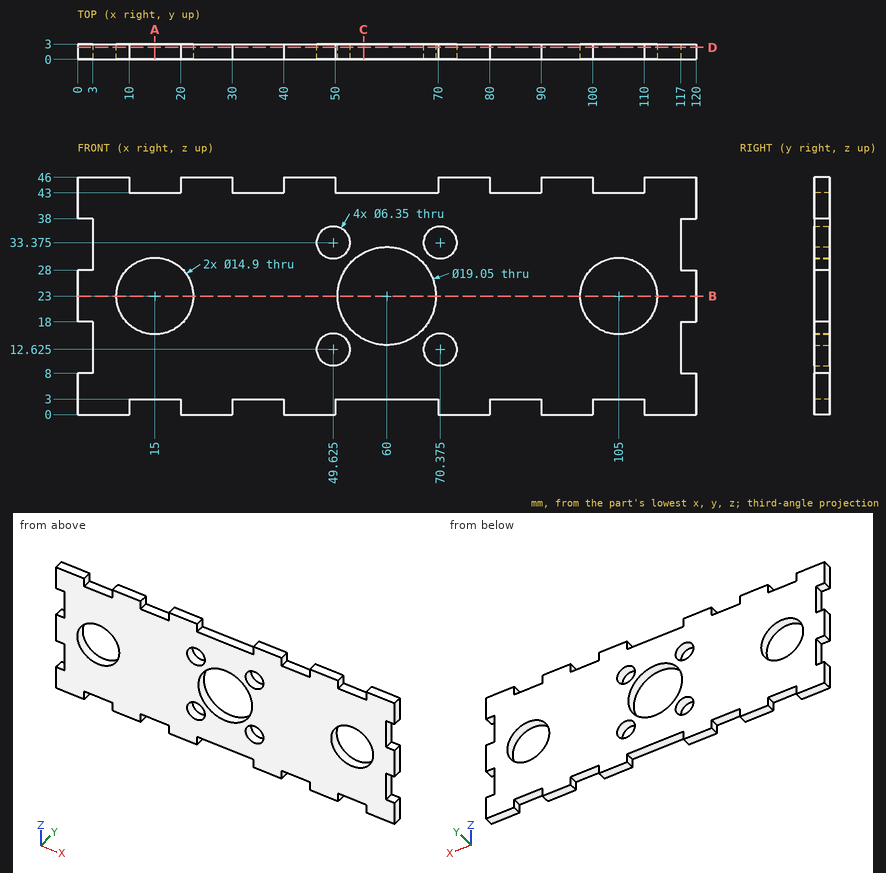
Drawing for the job (mm, zero at the part's lowest x, y, z). Coordinates: 2 decimals unless noted, no trailing zeros. Order: outer loops, then holes, each group sorted by start corner. A loop starts at its lowest first (then second) coordinate and runs counter-clockwise, first axis right, second up. Notation, with made-up numbers: (85, 66) -> (103, 66) arc R34 cw to (103, 102) -> close; hole circle Ø8 at (22.25, -3.5). An arc over 180 degrees is marked (long way). Return JSON: item names as keys, results as strings.
Item 1: Wall check: line 1 along X through (y, z) = (0.9, 23.5); line 2 along Z through (x, y) = (15, 1.1); line 3 along X through (y, z) = (1.45, 17.5). Give the ranges that are in metal, low to high. Write a range as from..to.
Model answer:
{"line 1": "x = 0..7.57, 22.43..50.49, 69.51..97.57, 112.43..120", "line 2": "z = 3..15.55, 30.45..43", "line 3": "x = 3..9.97, 20.03..52.22, 67.78..99.97, 110.03..117"}
Item 2: Slice it at B-B (z = 23). Write the cut outline in (x, y) (3 decimals), then the cut area to 3 significant figures.
Model answer:
{"outline": "(0, 0) -> (7.55, 0) -> (7.55, 3) -> (0, 3) -> close; (22.45, 0) -> (50.475, 0) -> (50.475, 3) -> (22.45, 3) -> close; (69.525, 0) -> (97.55, 0) -> (97.55, 3) -> (69.525, 3) -> close; (112.45, 0) -> (120, 0) -> (120, 3) -> (112.45, 3) -> close", "area": "213 mm²"}
Item 3: Pin check, flat tips, straight feed: P1, Ø1.5, axis at y = 1.5, z = 11.5, coming from the -X side; P2, Ø1.5, axis at x = 33, y = 1, coming from the -Z side; P3, Ø1, axis at y = 0.5, z = 13.5, coming from the +X side. Stop position of each tip, or through.
Model answer:
{"P1": "stops at x = 3", "P2": "stops at z = 3", "P3": "stops at x = 117"}
Item 4: Slice it at C-C (x = 55.5). Write the cut outline in (y, z), then the cut area to 3 significant figures.
Model answer:
{"outline": "(0, 3) -> (3, 3) -> (3, 14.61) -> (0, 14.61) -> close; (0, 31.39) -> (3, 31.39) -> (3, 43) -> (0, 43) -> close", "area": "69.6 mm²"}
Item 5: Slice it at D-D (y = 2.35). Count the separate pieces of the cut face and the enclosed holes in it, then the cut area to 3 significant figures.
Model answer:
{"separate pieces": "1", "enclosed holes": "7", "area": "4,280 mm²"}
Item 6: Slice it at A-A (x = 15). Write the cut outline in (y, z), then the cut area to 3 significant figures.
Model answer:
{"outline": "(0, 3) -> (3, 3) -> (3, 15.55) -> (0, 15.55) -> close; (0, 30.45) -> (3, 30.45) -> (3, 43) -> (0, 43) -> close", "area": "75.3 mm²"}
